from build123d import *

# Parameters (mm, degrees)
SKETCH1_W                     = 278.2
SKETCH1_H                     = 193.2
SHELL_BLOCK_DEPTH             = 27
SKETCH2_W                     = 273.2
SKETCH2_H                     = 185.8
FRONT_OPENING_DEPTH           = 1.5
SKETCH3_W                     = 273.2
SKETCH3_H                     = 188.2
DISPLAY_POCKET_DEPTH          = 22.5
SKETCH4_W                     = 3
SKETCH4_H                     = 56
VENT_SLOTS_DEPTH              = 4
SKETCH5_W                     = 58
SKETCH5_H                     = 16
CABLE_EXIT_X_SHORT_SIDE_DEPTH = 140.1
SKETCH6_R                     = 1.7
BOLT_HOLES_DEPTH              = 4


with BuildPart() as part:
    # Sketch1 → Shell Block (new body)
    with BuildSketch(Plane(origin=(0, 0, 0), x_dir=(1, 0, 0), z_dir=(0, 1, 0))):
        Rectangle(SKETCH1_W, SKETCH1_H)
    extrude(amount=SHELL_BLOCK_DEPTH)

    # Sketch2 → Front Opening (cut)
    with BuildSketch(Plane(origin=(0, 27, 0), x_dir=(1, 0, 0), z_dir=(0, 1, 0))):
        Rectangle(SKETCH2_W, SKETCH2_H)
    extrude(amount=-FRONT_OPENING_DEPTH, mode=Mode.SUBTRACT)

    # Sketch3 → Display Pocket (cut)
    with BuildSketch(Plane(origin=(0, 25.5, 0), x_dir=(1, 0, 0), z_dir=(0, 1, 0))):
        Rectangle(SKETCH3_W, SKETCH3_H)
    extrude(amount=-DISPLAY_POCKET_DEPTH, mode=Mode.SUBTRACT)

    # Sketch4 → Vent Slots (cut)
    with BuildSketch(Plane(origin=(0, 3, 0), x_dir=(1, 0, 0), z_dir=(0, 1, 0))):
        with Locations((-67.5, 56)):
            Rectangle(SKETCH4_W, SKETCH4_H)
        with Locations((-67.5, -56)):
            Rectangle(SKETCH4_W, SKETCH4_H)
        with Locations((-75.5, 56)):
            Rectangle(SKETCH4_W, SKETCH4_H)
        with Locations((-75.5, -56)):
            Rectangle(SKETCH4_W, SKETCH4_H)
        with Locations((-83.5, 56)):
            Rectangle(SKETCH4_W, SKETCH4_H)
        with Locations((-83.5, -56)):
            Rectangle(SKETCH4_W, SKETCH4_H)
        with Locations((-91.5, 56)):
            Rectangle(SKETCH4_W, SKETCH4_H)
        with Locations((-91.5, -56)):
            Rectangle(SKETCH4_W, SKETCH4_H)
        with Locations((-99.5, 56)):
            Rectangle(SKETCH4_W, SKETCH4_H)
        with Locations((-99.5, -56)):
            Rectangle(SKETCH4_W, SKETCH4_H)
        with Locations((-107.5, 56)):
            Rectangle(SKETCH4_W, SKETCH4_H)
        with Locations((-107.5, -56)):
            Rectangle(SKETCH4_W, SKETCH4_H)
        with Locations((-115.5, 56)):
            Rectangle(SKETCH4_W, SKETCH4_H)
        with Locations((-115.5, -56)):
            Rectangle(SKETCH4_W, SKETCH4_H)
        with Locations((-123.5, 56)):
            Rectangle(SKETCH4_W, SKETCH4_H)
        with Locations((-123.5, -56)):
            Rectangle(SKETCH4_W, SKETCH4_H)
    extrude(amount=-VENT_SLOTS_DEPTH, mode=Mode.SUBTRACT)

    # Sketch5 → Cable Exit (-X short side) (cut)
    with BuildSketch(Plane(origin=(0, 0, 0), x_dir=(0, 0, -1), z_dir=(1, 0, 0))):
        with Locations((0, 13)):
            Rectangle(SKETCH5_W, SKETCH5_H)
    extrude(amount=-CABLE_EXIT_X_SHORT_SIDE_DEPTH, mode=Mode.SUBTRACT)

    # Sketch6 → Bolt Holes (cut)
    with BuildSketch(Plane(origin=(0, 3, 0), x_dir=(1, 0, 0), z_dir=(0, 1, 0))):
        with Locations(Location((-40, -45, 0), (0, 0, 270))):
            Circle(SKETCH6_R)
        with Locations(Location((-40, 45, 0), (0, 0, 270))):
            Circle(SKETCH6_R)
        with Locations(Location((40, -45, 0), (0, 0, 270))):
            Circle(SKETCH6_R)
        with Locations(Location((40, 45, 0), (0, 0, 270))):
            Circle(SKETCH6_R)
        with Locations(Location((-52, -15, 0), (0, 0, 270))):
            Circle(SKETCH6_R)
        with Locations(Location((-52, 15, 0), (0, 0, 270))):
            Circle(SKETCH6_R)
        with Locations(Location((52, -15, 0), (0, 0, 270))):
            Circle(SKETCH6_R)
        with Locations(Location((52, 15, 0), (0, 0, 270))):
            Circle(SKETCH6_R)
        with Locations(Location((-12, -82, 0), (0, 0, 270))):
            Circle(SKETCH6_R)
        with Locations(Location((-12, 82, 0), (0, 0, 270))):
            Circle(SKETCH6_R)
        with Locations(Location((12, -82, 0), (0, 0, 270))):
            Circle(SKETCH6_R)
        with Locations(Location((12, 82, 0), (0, 0, 270))):
            Circle(SKETCH6_R)
        with Locations(Location((-124, -12, 0), (0, 0, 270))):
            Circle(SKETCH6_R)
        with Locations(Location((-124, 12, 0), (0, 0, 270))):
            Circle(SKETCH6_R)
        with Locations(Location((124, -12, 0), (0, 0, 270))):
            Circle(SKETCH6_R)
        with Locations(Location((124, 12, 0), (0, 0, 270))):
            Circle(SKETCH6_R)
        with Locations(Location((-72, 12, 0), (0, 0, 270))):
            Circle(SKETCH6_R)
        with Locations(Location((-72, -12, 0), (0, 0, 270))):
            Circle(SKETCH6_R)
    extrude(amount=-BOLT_HOLES_DEPTH, mode=Mode.SUBTRACT)


solid = part.part
Build history of the part. All positions in model axes, mm. A direction names the side the tool comes from. Coordinates: 2 decimals unless noted, no trailing zeros. Write each loop counter-clockwise with the first axis right and the second up, starting at its lowest first coordinate (ties: lowest second). Pieces come first, ordered by that corner, then holes.
(1) Cut at C-C on y = 15.5. List the corners of the cut face in (x, z), and give its area (3 significant figures).
(2) 3-axis set-ups, long thin cutter, end or side, ignore diameter. For faces 4 (the flat face through (-2, 14, -94.1)), 5 (the flat face through (-139.1, 22, 1)): which of +Z, -Z, +X, -X, +Y, -Y reach the whole face in a straight line?
(3) Drill centre lines: line 1 (Z direction, x = 124, y = 1.05); line 2 (X direction, y = 0.95, z = 15); line 3 (Z direction, x = -51, y = 10.5). Where is each one in solid material? Low to high.
(4) Cut at B-B on z = -32. State how many separate pieces and enclosed holes the cut face has, and give its area (3 significant figures).
(5) Mould opens along X. For faces 1 (the flat face through (-2, 14, 94.1)), 2 (the flat face through (139.1, 13, 1)), 3 (the flat face through (-2, 13, 96.6)) say: pulls with the +X half, pulls with the -X half, needs draft (parallel to the pull), parting line crosses it, or undercut.
(6) Cut at A-A on x = -7. List the corners of the cut face in (y, z), and give its area (3 significant figures).
(7) Pin check, flat tip, straight feed: pin 1 Ø5 at (x, z) = (-9.5, -20) entering from +Y. Stop position of the tip, or through.
Working result:
1. outline: (-139.1, -96.6) - (139.1, -96.6) - (139.1, 96.6) - (-139.1, 96.6) - (-139.1, 29) - (-136.6, 29) - (-136.6, 94.1) - (136.6, 94.1) - (136.6, -94.1) - (-136.6, -94.1) - (-136.6, -29) - (-139.1, -29) - close
1. area: 2,190 mm2
2. face 4: none
2. face 5: +Z, -Z, -X, +Y, -Y
3. line 1: z = -96.6 to -13.7, -10.3 to 10.3, 13.7 to 96.6
3. line 2: x = -139.1 to -53.7, -50.3 to 50.3, 53.7 to 139.1
3. line 3: z = -96.6 to -94.1, 94.1 to 96.6
4. separate pieces: 9
4. enclosed holes: 0
4. area: 883 mm2
5. face 1: undercut
5. face 2: pulls with the +X half
5. face 3: needs draft
6. outline: (0, -96.6) - (27, -96.6) - (27, -92.9) - (25.5, -92.9) - (25.5, -94.1) - (3, -94.1) - (3, 94.1) - (25.5, 94.1) - (25.5, 92.9) - (27, 92.9) - (27, 96.6) - (0, 96.6) - close
6. area: 703 mm2
7. pin 1: stops at y = 3
